```python
from build123d import *

# Parameters (mm, degrees)
BOSS_EXTRUDE1_DEPTH = 2
BOSS_EXTRUDE2_DEPTH = 4
SKETCH1_4_R         = 1.7
CUT_EXTRUDE1_DEPTH  = 10


with BuildPart() as part:
    # Sketch1 → Boss-Extrude1 (new body)
    with BuildSketch(Plane.XY):
        with BuildLine():
            Line((28.78011557, -21.498473491), (21.333027704, -14.051385626))
            ThreePointArc((21.333027704, -14.051385626), (20.684181007, -13.617840123), (19.918814142, -13.465599188))
            Line((19.918814142, -13.465599188), (-4.3, -13.465599188))
            ThreePointArc((-4.3, -13.465599188), (-6.421320344, -14.344278845), (-7.3, -16.465599188))
            Line((-7.3, -16.465599188), (-7.3, -99.073599188))
            ThreePointArc((-7.3, -99.073599188), (-6.421320344, -101.194919532), (-4.3, -102.073599188))
            Line((-4.3, -102.073599188), (19.918814142, -102.073599188))
            ThreePointArc((19.918814142, -102.073599188), (20.684181007, -101.921358253), (21.333027704, -101.48781275))
            Line((21.333027704, -101.48781275), (28.78511557, -94.035724885))
            ThreePointArc((28.78511557, -94.035724885), (32.741782732, -91.39196441), (37.408989873, -90.463599188))
            Line((37.408989873, -90.463599188), (107.834, -90.463599188))
            ThreePointArc((107.834, -90.463599188), (108.841627163, -90.046226351), (109.259, -89.038599188))
            Line((109.259, -89.038599188), (109.259, -26.495599188))
            ThreePointArc((109.259, -26.495599188), (108.841627163, -25.487972025), (107.834, -25.070599188))
            Line((107.834, -25.070599188), (37.403989873, -25.070599188))
            ThreePointArc((37.403989873, -25.070599188), (32.736782732, -24.142233967), (28.78011557, -21.498473491))
        make_face()
    extrude(amount=BOSS_EXTRUDE1_DEPTH)

    # Sketch1<3> → Boss-Extrude2 (add)
    with BuildSketch(Plane.XY):
        with BuildLine():
            Line((3, -16.169599188), (15.815448907, -16.169599188))
            ThreePointArc((15.815448907, -16.169599188), (18.129279051, -19.785919074), (22.322528351, -18.864919746))
            Line((22.322528351, -18.864919746), (31.232207794, -27.774599188))
            Line((31.232207794, -27.774599188), (102.655958934, -27.774599188))
            ThreePointArc((102.655958934, -27.774599188), (103.75222825, -30.577370938), (106.555, -31.673640255))
            Line((106.555, -31.673640255), (106.555, -83.860558122))
            ThreePointArc((106.555, -83.860558122), (103.75222825, -84.956827438), (102.655958934, -87.759599188))
            Line((102.655958934, -87.759599188), (31.237207794, -87.759599188))
            Line((31.237207794, -87.759599188), (22.322528351, -96.674278631))
            ThreePointArc((22.322528351, -96.674278631), (18.129279051, -95.753279303), (15.815448907, -99.369599188))
            Line((15.815448907, -99.369599188), (3, -99.369599188))
            ThreePointArc((3, -99.369599188), (1.51507576, -98.754523429), (0.9, -97.269599188))
            Line((0.9, -97.269599188), (0.9, -18.269599188))
            ThreePointArc((0.9, -18.269599188), (1.51507576, -16.784674948), (3, -16.169599188))
        make_face()
        with BuildLine():
            ThreePointArc((3, -17.969599188), (2.787867966, -18.057467154), (2.7, -18.269599188))
            Line((2.7, -18.269599188), (2.7, -42.574599188))
            Line((2.7, -42.574599188), (22, -42.574599188))
            Line((22, -42.574599188), (90.115, -42.574599188))
            Line((90.115, -42.574599188), (104.755, -42.574599188))
            Line((104.755, -42.574599188), (104.755, -33.225486399))
            ThreePointArc((104.755, -33.225486399), (102.479436044, -31.850163144), (101.104112789, -29.574599188))
            Line((101.104112789, -29.574599188), (30.486623382, -29.574599188))
            Line((30.486623382, -29.574599188), (22.147057077, -21.235032884))
            ThreePointArc((22.147057077, -21.235032884), (17.440448873, -21.448902232), (14.263602762, -17.969599188))
            Line((14.263602762, -17.969599188), (3, -17.969599188))
        make_face(mode=Mode.SUBTRACT)
        with BuildLine():
            ThreePointArc((2.7, -97.269599188), (2.787867966, -97.481731222), (3, -97.569599188))
            Line((3, -97.569599188), (14.263602762, -97.569599188))
            ThreePointArc((14.263602762, -97.569599188), (17.440448873, -94.090296144), (22.147057077, -94.304165492))
            Line((22.147057077, -94.304165492), (30.491623382, -85.959599188))
            Line((30.491623382, -85.959599188), (101.104112789, -85.959599188))
            ThreePointArc((101.104112789, -85.959599188), (102.479436044, -83.684035232), (104.755, -82.308711977))
            Line((104.755, -82.308711977), (104.755, -71.279599188))
            Line((104.755, -71.279599188), (90.115, -71.279599188))
            Line((90.115, -71.279599188), (22, -71.279599188))
            Line((22, -71.279599188), (2.7, -71.279599188))
            Line((2.7, -71.279599188), (2.7, -97.269599188))
        make_face(mode=Mode.SUBTRACT)
        Polygon((22, -69.479599188), (2.7, -69.479599188), (2.7, -44.374599188), (22, -44.374599188), (90.115, -44.374599188), (104.755, -44.374599188), (104.755, -69.479599188), (90.115, -69.479599188), align=None, mode=Mode.SUBTRACT)
    extrude(amount=-BOSS_EXTRUDE2_DEPTH)

    # Sketch1<4> → Cut-Extrude1 (cut)
    with BuildSketch(Plane.XY):
        with Locations((106.406, -27.923599188)):
            Circle(SKETCH1_4_R)
        with Locations((106.406, -87.610599188)):
            Circle(SKETCH1_4_R)
        with Locations((19.565489973, -99.220599188)):
            Circle(SKETCH1_4_R)
        with Locations((-4.447, -99.220599188)):
            Circle(SKETCH1_4_R)
        with Locations((-4.447, -16.318599188)):
            Circle(SKETCH1_4_R)
        with Locations((19.565489973, -16.318599188)):
            Circle(SKETCH1_4_R)
    extrude(amount=CUT_EXTRUDE1_DEPTH, mode=Mode.SUBTRACT)


solid = part.part
```
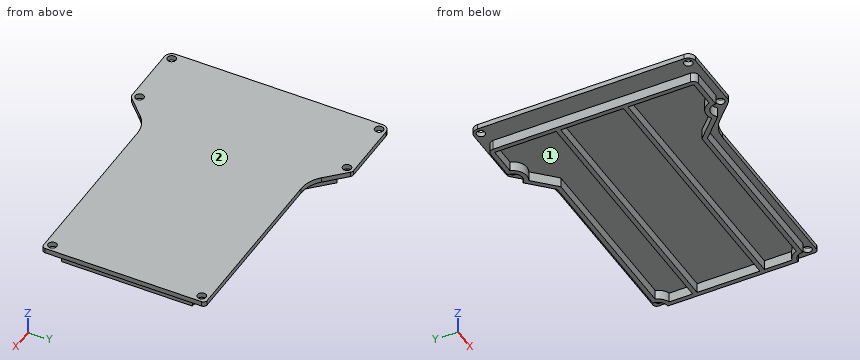
CAD build for the part. Positions are in the model's coordinates, mm. Face numbers are marked on the shaded views. Coordinates: 2 decimals unless noted, no trailing zeros. Order: outer loops, then holes, each group sorted by start corner. A loop starts at its lowest first (then second) coordinate and runs counter-clockwise, first axis right, second up. Notation, with made-up numbers: M 3.25,19 L 60.25,19 A16 ccw 60.25,40 Z; hole C 78,-5 d6. An arc over 180 degrees is marked long. Write each question's results on one line, items separated by ' | '. Start each with the question number.
Q1. Cut at A-A (y = -67.5). List the corners of the cut face in (x, z) (3 decimals).
Q2. Cut at C-C (z = 0.9). List the corners of the cut face in (x, y) (3 decimals).
Q3. Cut at D-D (x = 40). List the corners of the cut face in (y, z).
Q4. Pull direction X, two halves, no side cores. Call the marked faces 1 and 2: +X half, -X half, draft (parallel to the pull), parting line (faces both ways), or undercut.
Q5. Drill centre lines: probe 1 along Y at (x, z) = (71, -2.4); probe 2 along Y at (x, z) = (10.5, -2.35); probe 3 along X at (y, z) = (-79, -2.3) (3 decimals). Where is each one in solid material? Low to high. Write a range as from..to.
Q6. Flat gauge pins, fed straight in: P1, Ø0.6, axis at x = 89, z = 1, coming from the +Y side; P2, Ø2, axis at y = -34, z = -1.5, coming from the +X side (3 decimals); P3, Ø1.2, axis at y = -58, z = -3, coming from the -X side. Where does each tip first touch, or does it go through?
Q7. Cut at B-B (x = 10). List the corners of the cut face in (y, z), then the cut area to 3 significant figures.
Found:
1) outline: M -7.3,0 L 0.9,0 L 0.9,-4 L 2.7,-4 L 2.7,0 L 104.755,0 L 104.755,-4 L 106.555,-4 L 106.555,0 L 109.259,0 L 109.259,2 L -7.3,2 Z
2) outline: M -7.3,-99.074 A3 ccw -4.3,-102.074 L 19.919,-102.074 A2 ccw 21.333,-101.488 L 28.785,-94.036 A12.196 cw 37.409,-90.464 L 107.834,-90.464 A1.425 ccw 109.259,-89.039 L 109.259,-26.496 A1.425 ccw 107.834,-25.071 L 37.404,-25.071 A12.196 cw 28.78,-21.498 L 21.333,-14.051 A2 ccw 19.919,-13.466 L -4.3,-13.466 A3 ccw -7.3,-16.466 Z; hole C -4.447,-99.221 d3.4; hole C -4.447,-16.319 d3.4; hole C 19.565,-99.221 d3.4; hole C 19.565,-16.319 d3.4; hole C 106.406,-87.611 d3.4; hole C 106.406,-27.924 d3.4
3) outline: M -90.46,0 L -87.76,0 L -87.76,-4 L -85.96,-4 L -85.96,0 L -71.28,0 L -71.28,-4 L -69.48,-4 L -69.48,0 L -44.37,0 L -44.37,-4 L -42.57,-4 L -42.57,0 L -29.57,0 L -29.57,-4 L -27.77,-4 L -27.77,0 L -25.07,0 L -25.07,2 L -90.46,2 Z
4) face 1: undercut | face 2: draft
5) probe 1: -87.76..-85.96, -71.28..-69.48, -44.37..-42.57, -29.57..-27.77 | probe 2: -99.37..-97.57, -71.28..-69.48, -44.37..-42.57, -17.97..-16.17 | probe 3: 0.9..2.7, 104.755..106.555
6) P1: y = -25.07 | P2: x = 106.555 | P3: x = 0.9
7) outline: M -102.07,0 L -99.37,0 L -99.37,-4 L -97.57,-4 L -97.57,0 L -71.28,0 L -71.28,-4 L -69.48,-4 L -69.48,0 L -44.37,0 L -44.37,-4 L -42.57,-4 L -42.57,0 L -17.97,0 L -17.97,-4 L -16.17,-4 L -16.17,0 L -13.47,0 L -13.47,2 L -102.07,2 Z | area: 206 mm²
